```python
from build123d import *

# Parameters (mm, degrees)
BOSS_EXTRU_1_DEPTH      = 10
BOSS_EXTRU_2_DEPTH      = 10
ESQUISSE3_R             = 3
ENL_V_MAT_EXTRU_1_DEPTH = 10


with BuildPart() as part:
    # Esquisse1 → Boss.-Extru.1 (new body)
    with BuildSketch(Plane.XY):
        with BuildLine():
            Line((0, 42), (0, 50))
            ThreePointArc((0, 50), (35.355339059, 35.355339059), (50, 0))
            Line((50, 0), (42, 0))
            ThreePointArc((42, 0), (29.69848481, 29.69848481), (0, 42))
        make_face()
    extrude(amount=BOSS_EXTRU_1_DEPTH)

    # Esquisse2 → Boss.-Extru.2 (add)
    with BuildSketch(Plane.XY.offset(10)):
        with BuildLine():
            Line((0, 42), (0, 50))
            ThreePointArc((0, 50), (-10.472135955, 46), (0, 42))
        make_face()
        with BuildLine():
            Line((42, 0), (50, 0))
            ThreePointArc((50, 0), (46, -10.472135955), (42, 0))
        make_face()
    extrude(amount=-BOSS_EXTRU_2_DEPTH)

    # Esquisse3 → Enlèv. mat.-Extru.1 (cut)
    with BuildSketch(Plane.XY.offset(10)):
        with Locations((46, -4.472135955)):
            Circle(ESQUISSE3_R)
        with Locations((-4.472135955, 46)):
            Circle(ESQUISSE3_R)
    extrude(amount=-ENL_V_MAT_EXTRU_1_DEPTH, mode=Mode.SUBTRACT)


solid = part.part
```
Geometry: final body of the model. Coordinates: model frame, mm. Give positions to 0.01 mm unless a question says otherwise; leave off trailing zeros. Loops run counter-clockwise (first coordinate to the right, second up) from the corner with the lowest first, then second, coordinate; pieces in that order, holes last. Notation, with made-up numbers: (-23, -6.75) -> (34, -6.75) arc R27 ccw to (34, 11.25) -> close; hole circle Ø7 at (68, 24). An arc over 180 degrees is marked (long way). Use CSV: the item, a comma, the result in double quotes.
(1) Cut plane A-A (x = 47.5). Output: boundary loops of the cut face in (y, z), plus the area to 3 significant figures.
From the geometry:
outline,"(-10.28, 0) -> (-7.07, 0) -> (-7.07, 10) -> (-10.28, 10) -> close; (-1.87, 0) -> (15.61, 0) -> (15.61, 10) -> (-1.87, 10) -> close"
area,"207 mm^2"
(2) Ray query, line 1 along Y through (x, z) = (-4.5, 7); line 2 along Y through (x, z) = (46, 5.25); line 3 along X through (y, z) = (45.5, 6.75). Return the intervals inside material, ascending. Write a range as [from, to].
From the geometry:
line 1,"[40, 43], [49, 52]"
line 2,"[-10.47, -7.47], [-1.47, 19.6]"
line 3,"[-10.45, -7.43], [-1.51, 20.73]"
(3) Cut plane B-B (y = 46). Output: boundary loops of the cut face in (x, z).
From the geometry:
outline,"(-10.47, 0) -> (-7.47, 0) -> (-7.47, 10) -> (-10.47, 10) -> close; (-1.47, 0) -> (19.6, 0) -> (19.6, 10) -> (-1.47, 10) -> close"
(4) Cut plane C-C (z = 2). Output: boundary loops of the cut face in (x, y).
From the geometry:
outline,"(0, 42) arc R42 cw to (42, 0) arc R6 ccw (long way) to (50, 0) arc R50 ccw to (0, 50) arc R6 ccw (long way) to start; hole circle Ø6 at (-4.47, 46); hole circle Ø6 at (46, -4.47)"
(5) Pull-direction query (X, two-part tool) for faces 1 (the face through (32, 28, 0)), 2 (the face through (46.2, -10.47, 5.07)), 3 (the face through (-10.47, 46.2, 5.07)), 4 (the face through (30.023, 29.37, 4.93)); classes: released by +X, released by -X, zero draft, split by the parting line, or undercut.
From the geometry:
face 1,"zero draft"
face 2,"split by the parting line"
face 3,"undercut"
face 4,"undercut"
(6) First-contact query: P1, Ø2, axis at x = 10, z = 3, coming from the -Y side; P2, Ø1, axis at y = 3.5, z = 9, coming from the -X side; P3, Ø9.5, axis at x = 46, y = -4.47, coming from the +Z side; P4, Ø3, axis at y = 15.5, z = 2, coming from the +X side. Flat tips, straight axial feed; report the tip coordinate or a pass-through.
From the geometry:
P1,"y = 40.53"
P2,"x = 41.81"
P3,"z = 10"
P4,"x = 48"
(7) Cut plane D-D (y = 32.5). Output: boundary loops of the cut face in (x, z).
From the geometry:
outline,"(26.6, 0) -> (38, 0) -> (38, 10) -> (26.6, 10) -> close"
